Here's the drawing with two shaded views (mm, measured from the low corner). I have some questions. Give positions to 0.01 mm unless a question says otherwise; leave off trailing zeros. Write each loop counter-clockwise with the first axis right and the second up, starting at its lowest first coordinate (ties: lowest second). Pieces come first, ordered by that corner, then holes. Notation, with made-up numbers: M 49.5,-23.5 L 87.5,-23.5 A23 ccw 87.5,-9.5 Z; hole C 49.25,66 d2. An arc over 180 degrees is marked long. Use one line per item in the form item = value.
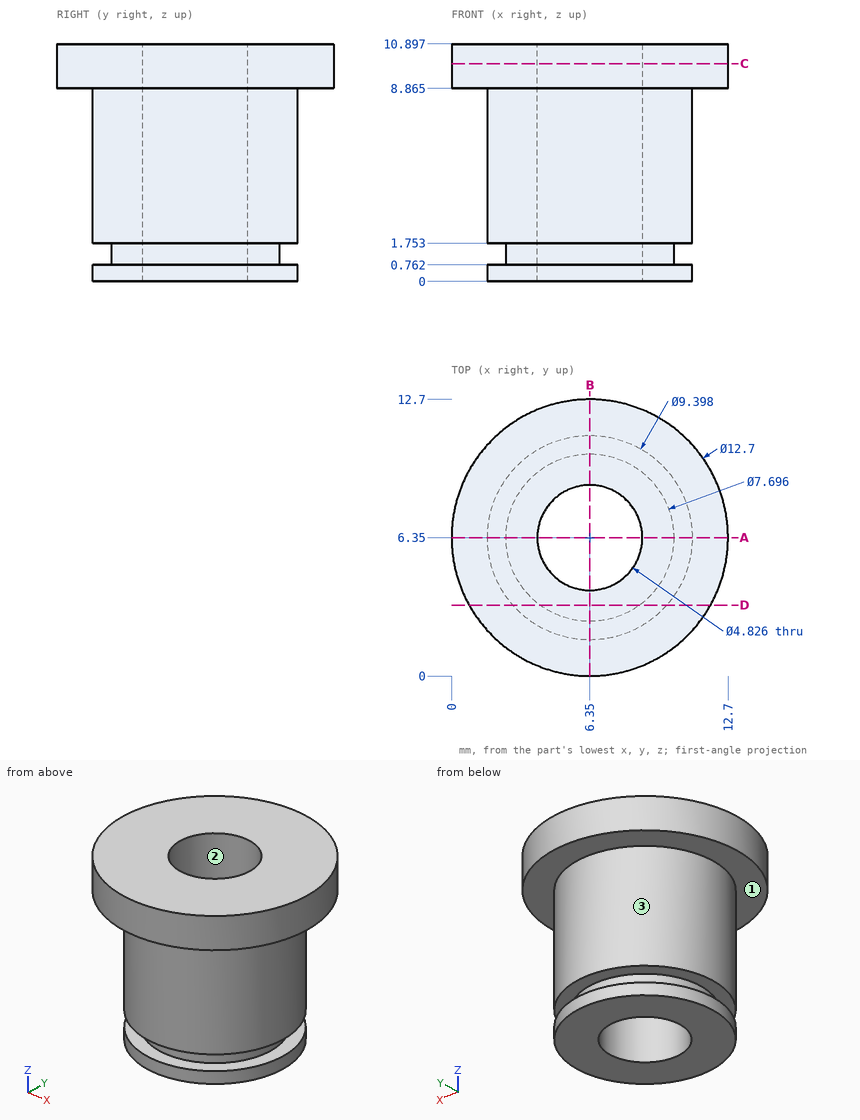
1) Thinking about a two-plate mould opening in X: for the marked faces 1, 2 and 3, which applies, released by +X, released by -X, zero draft, split by the parting line, or undercut?
Checked values:
face_1 = zero draft
face_2 = undercut
face_3 = split by the parting line
2) For pin 1 Ø4 at (x, y) = (7.5, 7.5) entering from +Z; pin 2 Ø5 at (x, z) = (5.5, 1.5) entering from +Y; pin 3 Ø1 at (y, z) = (5, 9.5) entering from -X, each with a flat end and sliding along its axis, tell me the tip position at first contact or that it passes through.
Checked values:
pin_1 = 10.9
pin_2 = 11.05
pin_3 = 0.06
3) I want a section at C-C, the plane z = 10. Please give me the cut outline in (x, y), plus the area to 3 significant figures.
Checked values:
outline = C 6.35,6.35 d12.7; hole C 6.35,6.35 d4.83
area = 108 mm2
4) If I drill on L1, parallel to Z at x = 2.5, y = 5; L2, parallel to X at y = 6.25, z = 10.25; L3, parallel to Y at x = 6.35, z = 6, over which ranges is the centre line in solid material (lowest first)?
Checked values:
L1 = 0 to 0.76, 1.75 to 10.9
L2 = 0 to 3.94, 8.76 to 12.7
L3 = 1.65 to 3.94, 8.76 to 11.05
5) I want a section at A-A, the plane y = 6.35. Please give me the cut outline in (x, z) (1 decimal).
Checked values:
outline = M 0,8.9 L 1.7,8.9 L 1.7,1.8 L 2.5,1.8 L 2.5,0.8 L 1.7,0.8 L 1.7,0 L 3.9,0 L 3.9,10.9 L 0,10.9 Z; M 8.8,0 L 11,0 L 11,0.8 L 10.2,0.8 L 10.2,1.8 L 11,1.8 L 11,8.9 L 12.7,8.9 L 12.7,10.9 L 8.8,10.9 Z
6) I want a section at D-D, the plane y = 3.25. Please give me the cut outline in (x, z) (1 decimal).
Checked values:
outline = M 0.8,8.9 L 2.8,8.9 L 2.8,1.8 L 4.1,1.8 L 4.1,0.8 L 2.8,0.8 L 2.8,0 L 9.9,0 L 9.9,0.8 L 8.6,0.8 L 8.6,1.8 L 9.9,1.8 L 9.9,8.9 L 11.9,8.9 L 11.9,10.9 L 0.8,10.9 Z
